Here's how the part is built. I have some questions about the finished solid (model axes, mm). A direction names the side the tool comes from. Coordinates: 2 decimals unless noted, no trailing zeros. Write each loop counter-clockwise with the first axis right and the second up, starting at its lowest first coordinate (ties: lowest second). Pieces come first, ordered by that corner, then holes. Notation, with made-up numbers: (10.5, -38.5) -> (32.5, -38.5) arc R27 cw to (32.5, -4.5) -> close; hole circle Ø1 at (-3, -26.5). An arc over 180 degrees is marked (long way). Put each result on its own line as item: value. Start each with the question number.
Item 1: I need wall thicknesses on line 1 (Y direction, x = 2.9, z = 8.5); line 2 (Z direction, x = 3.4, y = 3.5); line 3 (Z direction, x = 1, y = -1.25). Which ranges of each line are inside material? Lowest first, please. Write a range as [from, to].
Item 2: I want a section at B-B, the plane x = 1.6. List the corners of the cut face in (y, z) for me.
Item 3: I want a section at D-D, the plane z = -37. List the corners of the cut face in (x, y) for me.
Item 4: For pin 1 (2 mm diameter, centred on x = 4.5, y = 5, fed in from +Z); pin 2 (2 mm diameter, centred on y = -1, z = -16, fed in from -X); pin 3 (3 mm diameter, centred on x = 2.5, y = -6.5, fed in from +Z), each with a flat end and sliding along its axis, tell me the tip position at first contact or that it passes through.
Item 5: On a 3-axis mill with a long thin cutter (end or side, diameter ignored), from which of +Z, -Z, +X, -X, +Y, -Y can I reach the whole of each face in a straight line? I mean faces 4 (the face through (3, 4, 18)), 5 (the face through (5, -4.3, -0.6)). Say none if no direction works.
Item 6: If we mould it in two halves opening along Y, with no side actions, what happens to faces 1 (the face through (3, -4, 17)), 2 (the face through (2, -10, 0)), 3 (the face through (2, 0, 45))? For each: released by +Y, released by -Y, zero draft, split by the parting line, or undercut.
Item 7: I want a section at C-C, the plane z = 29. List the corners of the cut face in (x, y) for me.
Item 8: I want a section at A-A, the plane y = 0. List the corners of the cut face in (x, z) for me, then the cut area to 3 significant figures.
from build123d import *

# Parameters (mm, degrees)
BOSS_EXTRUDE1_DEPTH = 5
SKETCH2_R           = 4
SKETCH2_R_2         = 3
CUT_EXTRUDE1_DEPTH  = 6


with BuildPart() as part:
    # Sketch1 → Boss-Extrude1 (new body)
    with BuildSketch(Plane(origin=(0, 0, 0), x_dir=(0, 0, -1), z_dir=(1, 0, 0))):
        with BuildLine():
            Line((-35, 10), (35, 10))
            ThreePointArc((35, 10), (45, 0), (35, -10))
            Line((35, -10), (-35, -10))
            ThreePointArc((-35, -10), (-45, 0), (-35, 10))
        make_face()
    extrude(amount=BOSS_EXTRUDE1_DEPTH)

    # Sketch2 → Cut-Extrude1 (cut, through all)
    with BuildSketch(Plane(origin=(5, 0, 0), x_dir=(0, 0, -1), z_dir=(1, 0, 0))):
        with Locations((17, 0)):
            Circle(SKETCH2_R)
        with Locations((37, 0)):
            Circle(SKETCH2_R_2)
        with BuildLine():
            Line((-35, 4), (0, 4))
            ThreePointArc((0, 4), (4, 0), (0, -4))
            Line((0, -4), (-35, -4))
            ThreePointArc((-35, -4), (-39, 0), (-35, 4))
        make_face()
    extrude(amount=-CUT_EXTRUDE1_DEPTH, mode=Mode.SUBTRACT)


solid = part.part
Calculated:
1. line 1: y = [-10, -4], [4, 10]
1. line 2: z = [-44.37, -18.94], [-15.06, -1.94], [36.94, 44.37]
1. line 3: z = [-44.92, -39.73], [-34.27, -20.8], [-13.2, -3.8], [38.8, 44.92]
2. outline: (-10, -35) arc R10 ccw to (10, -35) -> (10, 35) arc R10 ccw to (-10, 35) -> close; hole circle Ø8 at (0, -17); hole (-4, 0) arc R4 ccw to (4, 0) -> (4, 35) arc R4 ccw to (-4, 35) -> close; hole circle Ø6 at (0, -37)
3. outline: (0, -9.8) -> (5, -9.8) -> (5, -3) -> (0, -3) -> close; (0, 3) -> (5, 3) -> (5, 9.8) -> (0, 9.8) -> close
4. pin 1: stops at z = 44.17
4. pin 2: passes through
4. pin 3: stops at z = 43.66
5. face 4: +X, -X
5. face 5: +Z, -Z, +X, +Y, -Y
6. face 1: undercut
6. face 2: released by -Y
6. face 3: split by the parting line
7. outline: (0, -10) -> (5, -10) -> (5, -4) -> (0, -4) -> close; (0, 4) -> (5, 4) -> (5, 10) -> (0, 10) -> close
8. outline: (0, -45) -> (5, -45) -> (5, -40) -> (0, -40) -> close; (0, -34) -> (5, -34) -> (5, -21) -> (0, -21) -> close; (0, -13) -> (5, -13) -> (5, -4) -> (0, -4) -> close; (0, 39) -> (5, 39) -> (5, 45) -> (0, 45) -> close
8. area: 165 mm2
